The drawing under review shows one solid part. Ordinate dimensions are in mm from its lowest x, y, z. Give positions to 0.01 mm unless a question says otherwise; leave off trailing zeros. Order: outer loops, then holes, each group sorted by start corner. A loop starts at its lowest first (then second) coordinate and runs counter-clockwise, first axis right, second up. Notation, with made-up numbers: M 57,-24.75 L 102,-24.75 A36 ccw 102,13.25 Z; hole C 88,80 d11. An arc over 180 degrees is marked long. Put each result on its own line as item: value. Start each with the question number.
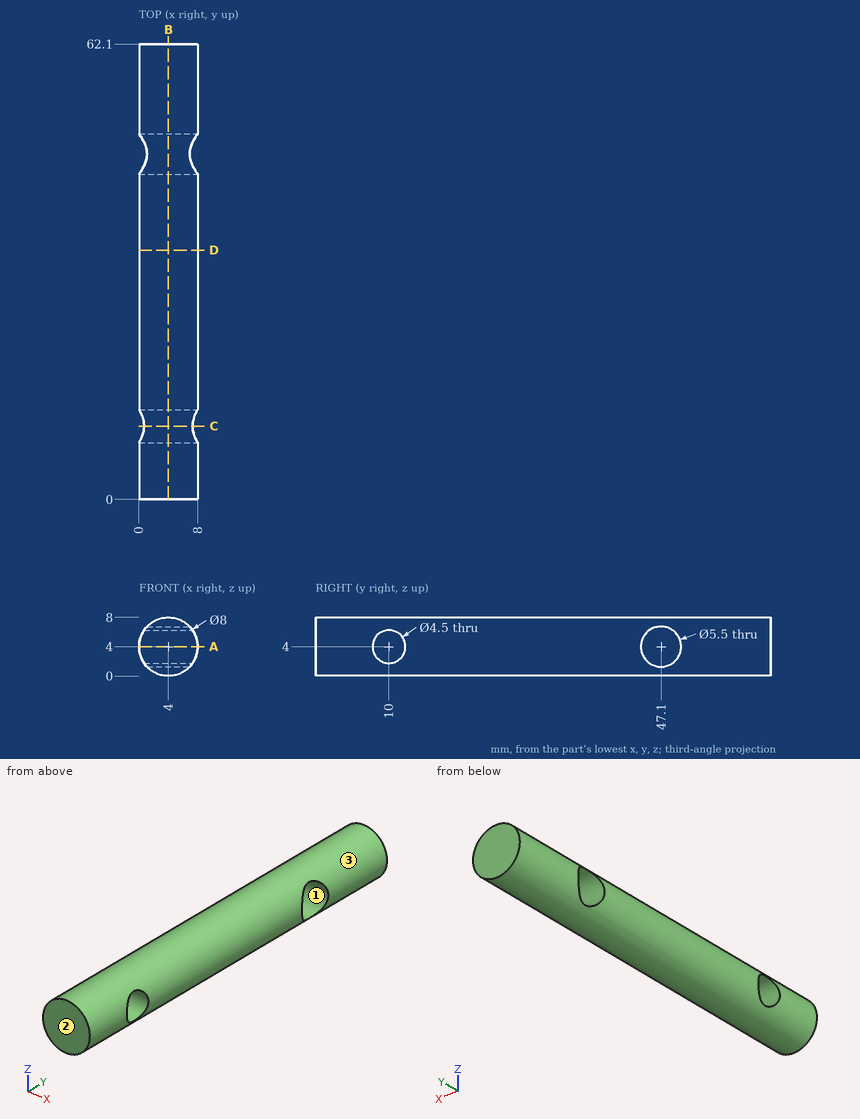
1. Insertion check: pin 1 (4 mm diameter, centred on y = 46.5, z = 2.5, fed in from +X); pin 2 (4 mm diameter, centred on y = 54, z = 2.5, fed in from +X); pin 3 (1.5 mm diameter, centred on x = 5, y = 52.5, fed in from -Z). Each pin has a flat end and moves straight along its axis. Give the tip position at first contact, or say it passes through.
2. Consider section C-C on y = 10. Give the boundary of the cut face in (x, z), then the cut area to 3 significant figures.
3. Consider section B-B on x = 4. Give the boundary of the cut face in (y, z).
4. Consider section A-A on z = 4. Give the boundary of the cut face in (x, y).
5. The part is to be moulded in two halves that separate along Z. For the marked faces 1, 2 and 3, say which applies: +Z half, -Z half, draft (parallel to the pull), parting line (faces both ways), or undercut.
6. Consider section D-D on y = 34. Give the boundary of the cut face in (x, z).
7. To check wall thickness, follow probe 1 along Y at (x, z) = (2.5, 4); probe 2 along Y at (x, z) = (7.5, 2.75); probe 3 along X at (y, z) = (24, 4.25). State the ranges of each line that lie inside material, in increasing order.
Returned:
1. pin 1: stops at x = 7.86
1. pin 2: stops at x = 8
1. pin 3: stops at z = 0.01
2. outline: M 0.69,1.75 A4 ccw 7.31,1.75 Z; M 0.69,6.25 L 7.31,6.25 A4 ccw Z
2. area: 16.3 mm2
3. outline: M 0,0 L 62.1,0 L 62.1,8 L 0,8 Z; hole C 10,4 d4.5; hole C 47.1,4 d5.5
4. outline: M 0,0 L 8,0 L 8,7.75 L 0,7.75 Z; M 0,12.25 L 8,12.25 L 8,44.35 L 0,44.35 Z; M 0,49.85 L 8,49.85 L 8,62.1 L 0,62.1 Z
5. face 1: undercut
5. face 2: draft
5. face 3: parting line
6. outline: C 4,4 d8
7. probe 1: y = 0 to 7.75, 12.25 to 44.35, 49.85 to 62.1
7. probe 2: y = 0 to 8.13, 11.87 to 44.65, 49.55 to 62.1
7. probe 3: x = 0.01 to 7.99
